from build123d import *

# Parameters (mm, degrees)
F0_R     = 50.8
F1_DEPTH = 7.14375
F3_DEPTH = 7.14475
F4_R     = 1.27
F5_R     = 4.7625
F6_DEPTH = 3.81


with BuildPart() as f1:
    # F0 (on Top) → F1 (new body)
    with BuildSketch(Plane.XY):
        Circle(F0_R)
        Polygon((-12.7582862486, 0), (-6.3791431243, 11.049), (6.3791431243, 11.049), (12.7582862486, 0), (6.3791431243, -11.049), (-6.3791431243, -11.049), align=None, mode=Mode.SUBTRACT)
    extrude(amount=F1_DEPTH)

    # F2 (on face) → F3 (cut, through all)
    with BuildSketch(Plane.XY.offset(7.14375)):
        with BuildLine():
            Line((-6.3791431243, -40.1362197149), (-6.3791431243, -27.8538535575))
            ThreePointArc((-6.3791431243, -27.8538535575), (-24.7466759131, -14.2875), (-27.3117163362, 8.4024267787))
            Line((-27.3117163362, 8.4024267787), (-37.9485574471, 14.5436098574))
            ThreePointArc((-37.9485574471, 14.5436098574), (-35.1952724098, -20.32), (-6.3791431243, -40.1362197149))
        make_face()
        Polygon((-38.3481822298, 25.019), (-40.8411806922, 25.019), (-42.0876799234, 22.86), (-40.8411806922, 20.701), (-38.3481822298, 20.701), (-37.1016829987, 22.86), align=None)
        Polygon((1.2464992312, -43.561), (-1.2464992312, -43.561), (-2.4929984624, -45.72), (-1.2464992312, -47.879), (1.2464992312, -47.879), (2.4929984624, -45.72), align=None)
        Polygon((40.8411806922, 25.019), (38.3481822298, 25.019), (37.1016829987, 22.86), (38.3481822298, 20.701), (40.8411806922, 20.701), (42.0876799234, 22.86), align=None)
        with BuildLine():
            ThreePointArc((-20.9325732119, 19.4514267787), (0, 28.575), (20.9325732119, 19.4514267787))
            Line((20.9325732119, 19.4514267787), (31.5694143228, 25.5926098574))
            ThreePointArc((31.5694143228, 25.5926098574), (0, 40.64), (-31.5694143228, 25.5926098574))
            Line((-31.5694143228, 25.5926098574), (-20.9325732119, 19.4514267787))
        make_face()
        with BuildLine():
            Line((6.3791431243, -27.8538535575), (6.3791431243, -40.1362197149))
            ThreePointArc((6.3791431243, -40.1362197149), (35.1952724098, -20.32), (37.9485574471, 14.5436098574))
            Line((37.9485574471, 14.5436098574), (27.3117163362, 8.4024267787))
            ThreePointArc((27.3117163362, 8.4024267787), (28.2574142422, 4.2484309276), (28.575, 0))
            ThreePointArc((28.575, 0), (22.3474231152, -17.8079562306), (6.3791431243, -27.8538535575))
        make_face()
        with BuildLine():
            Line((6.3791431243, -14.5369239525), (6.3791431243, -21.2898369651))
            ThreePointArc((6.3791431243, -21.2898369651), (17.8287279543, -13.2697808773), (22.225, 0))
            ThreePointArc((22.225, 0), (22.0750217642, 2.5776033652), (21.6271112163, 5.1204184825))
            Line((21.6271112163, 5.1204184825), (15.7789169979, 1.7439619762))
            ThreePointArc((15.7789169979, 1.7439619762), (15.8509610488, 0.8733034006), (15.875, 0))
            ThreePointArc((15.875, 0), (13.2906832424, -8.6817834545), (6.3791431243, -14.5369239525))
        make_face()
        with BuildLine():
            Line((9.3997738736, 12.7929619762), (15.2479680921, 16.1694184825))
            ThreePointArc((15.2479680921, 16.1694184825), (0, 22.225), (-15.2479680921, 16.1694184825))
            Line((-15.2479680921, 16.1694184825), (-9.3997738736, 12.7929619762))
            ThreePointArc((-9.3997738736, 12.7929619762), (0, 15.875), (9.3997738736, 12.7929619762))
        make_face()
        with BuildLine():
            ThreePointArc((-21.6271112163, 5.1204184825), (-19.2474145991, -11.1125), (-6.3791431243, -21.2898369651))
            Line((-6.3791431243, -21.2898369651), (-6.3791431243, -14.5369239525))
            ThreePointArc((-6.3791431243, -14.5369239525), (-13.7481532851, -7.9375), (-15.7789169979, 1.7439619762))
            Line((-15.7789169979, 1.7439619762), (-21.6271112163, 5.1204184825))
        make_face()
    extrude(amount=-F3_DEPTH, mode=Mode.SUBTRACT)

    # F4
    f4_edges = [f1.edges().sort_by_distance(p)[0] for p in [
        (-37.948557, 14.54361, 3.571875),
        (-27.311716, 8.402427, 3.571875),
        (-6.379143, -40.13622, 3.571875),
        (-6.379143, -27.853854, 3.571875),
        (-21.627111, 5.120418, 3.571875),
        (-15.778917, 1.743962, 3.571875),
        (-6.379143, -21.289837, 3.571875),
        (-6.379143, -14.536924, 3.571875),
        (6.379143, -21.289837, 3.571875),
        (6.379143, -14.536924, 3.571875),
        (21.627111, 5.120418, 3.571875),
        (15.778917, 1.743962, 3.571875),
        (6.379143, -40.13622, 3.571875),
        (6.379143, -27.853854, 3.571875),
        (37.948557, 14.54361, 3.571875),
        (27.311716, 8.402427, 3.571875),
        (31.569414, 25.59261, 3.571875),
        (20.932573, 19.451427, 3.571875),
        (-31.569414, 25.59261, 3.571875),
        (-20.932573, 19.451427, 3.571875),
        (15.247968, 16.169418, 3.571875),
        (9.399774, 12.792962, 3.571875),
        (-15.247968, 16.169418, 3.571875),
        (-9.399774, 12.792962, 3.571875),
    ]]
    fillet(f4_edges, radius=F4_R)

    # F5 (on face) → F6 (cut)
    with BuildSketch(Plane.XY.offset(7.14375)):
        with Locations((-39.594681461, 22.86)):
            Circle(F5_R)
        Polygon((-42.0876799234, 22.86), (-40.8411806922, 25.019), (-38.3481822298, 25.019), (-37.1016829987, 22.86), (-38.3481822298, 20.701), (-40.8411806922, 20.701), align=None, mode=Mode.SUBTRACT)
        with Locations((39.594681461, 22.86)):
            Circle(F5_R)
        Polygon((38.3481822298, 25.019), (40.8411806922, 25.019), (42.0876799234, 22.86), (40.8411806922, 20.701), (38.3481822298, 20.701), (37.1016829987, 22.86), align=None, mode=Mode.SUBTRACT)
        with Locations((0, -45.72)):
            Circle(F5_R)
        Polygon((-2.4929984624, -45.72), (-1.2464992312, -43.561), (1.2464992312, -43.561), (2.4929984624, -45.72), (1.2464992312, -47.879), (-1.2464992312, -47.879), align=None, mode=Mode.SUBTRACT)
    extrude(amount=-F6_DEPTH, mode=Mode.SUBTRACT)


solid = f1.part
For this review, take the finished solid that the model builds, in its own axes (mm). A direction names the side the tool comes from. Round coordinates to 2 decimals unless told otherwise and drop trailing zeros. Order: outer loops, then holes, each group sorted by start corner. A loop starts at its lowest first (then second) coordinate and runs counter-clockwise, first axis right, second up. Notation, with made-up numbers: M 40.5,-9.75 L 88.5,-9.75 A15 ccw 88.5,1.25 Z; hole C -32.5,76.25 d6. An arc over 180 degrees is marked long. Use a Markdown table: item, result. Add a question column.
Item 1: Insertion check: pin 1 (0.7 mm diameter, centred on x = 0, z = 1.5, fed in from -Y); pin 2 (3 mm diameter, centred on y = -27.5, z = 2.5, fed in from -X); pin 3 (0.7 mm diameter, centred on x = -39.5, z = 2, fed in from -Y); pin 4 (10 mm diameter, centred on x = -23, y = 1, fed in from -Z). Each pin has a flat end and moves straight along its axis. Give the tip position at first contact, or say it passes through.
Item 2: Add section B-B, the plane y = -16.5. Give the boundary of the cut face in (x, z), then the cut area to 3 significant figures.
Item 3: Mouldability with a two-part tool opening along X and no side actions: class faces 3 (the flat face through (-6.379, -17, 4)), 4 (the cylindrical face through (-11.012, -49.592, 3.522)) as released by +X, released by -X, zero draft, split by the parting line, or undercut.
Item 4: Add section C-C, the plane x = -33. Give the boundary of the cut face in (y, z), then the cut area to 3 significant figures.
Item 5: To check wall thickness, follow line 1 along Y through (x, z) = (0, 5.05) (1 decimal); line 2 along X through (y, z) = (-11, 3); line 3 along Y through (x, z) = (-12, 1.25). State the ranges of each line that lie inside material, in increasing order.
Item 6: Add section A-A, the plane x = 0. State how many separate pieces and enclosed holes the cut face has, then the cut area to 3 significant figures.
Item 7: Tool access review of faces 1 (the flat face through (42, 22, 3.334)), 2 (the flat face through (1.861, -46.815, 1.69)): name each direction out of +Z, -Z, +X, -X, +Y, -Y from which nothing blocks a thin tool from reaching the whole face with its end or side.
Geometry results:
| question | item | result |
|---|---|---|
| 1 | pin 1 | stops at y = -50.8 |
| 1 | pin 2 | stops at x = -43.64 |
| 1 | pin 3 | stops at y = -32.37 |
| 1 | pin 4 | stops at z = 0 |
| 2 | outline | M -48.05,0 L -37.14,0 L -37.14,7.14 L -48.05,7.14 Z; M -23.33,0 L -14.89,0 L -14.89,7.14 L -23.33,7.14 Z; M -6.38,0 L 6.38,0 L 6.38,7.14 L -6.38,7.14 Z; M 14.89,0 L 23.33,0 L 23.33,7.14 L 14.89,7.14 Z; M 37.14,0 L 48.05,0 L 48.05,7.14 L 37.14,7.14 Z |
| 2 | area | 368 mm² |
| 3 | face 3 | undercut |
| 3 | face 4 | split by the parting line |
| 4 | outline | M -38.62,0 L -23.72,0 L -23.72,7.14 L -38.62,7.14 Z; M 11.69,0 L 38.62,0 L 38.62,7.14 L 11.69,7.14 Z |
| 4 | area | 299 mm² |
| 5 | line 1 | y = -50.8 to -50.5, -41 to -11, 11 to 15.9, 22.2 to 28.6, 40.6 to 50.8 |
| 5 | line 2 | x = -49.59 to -39.12, -26.37 to -19.31, -11.45 to -6.41, 6.41 to 11.45, 19.31 to 26.37, 39.12 to 49.59 |
| 5 | line 3 | y = -49.36 to -38.83, -25.93 to -18.71, -10.39 to -1.31, 1.31 to 14.29, 18.71 to 25.93, 38.83 to 49.36 |
| 6 | separate pieces | 5 |
| 6 | enclosed holes | 0 |
| 6 | area | 386 mm² |
| 7 | face 1 | +Z |
| 7 | face 2 | +Z, -Z |
